Could you check a few things on this drawing? It's one solid part, dimensions in mm from its lowest x, y, z. Coordinates: 2 decimals unless noted, no trailing zeros. Write each loop counter-clockwise with the first axis right and the second up, starting at its lowest first coordinate (ties: lowest second). Pieces come first, ordered by that corner, then holes. Notation, with made-up numbers: (23, 16) - (38, 16) arc R23 cw to (38, 36) - close; hole circle Ø5 at (0, 58.5). An arc over 180 degrees is marked (long way). Answer as a JSON object with one key per item and string values. Group by question number.
1) If we section it at D-D (x = 12.75): Write out the boundary of the cut face in (y, z), plus the area to 3 significant figures.
2) Please list where these lines run through material, in increasing order: line 1 along Y through (x, z) = (4, 1.15); line 2 along Z through (x, y) = (3, 0.95); line 3 along Z through (x, y) = (6.75, 12).
3) If we section it at A-A (z = 26): Write out the boundary of the cut face in (x, y), plus the area to 3 significant figures.
4) If we section it at C-C (x = 4): Write out the boundary of the cut face in (y, z), plus the area to 3 significant figures.
5) Will these pins go through, and if not, where does the flat tip stop? pin 1 Ø2.5 at (x, y) = (16, 16) entering from +Z; pin 2 Ø5 at (x, z) = (13.5, 12) entering from -Y; pin 3 Ø10 at (x, z) = (13.5, 14.5) entering from +Y; pin 4 Ø9 at (x, y) = (9, 10.5) entering from +Z.
6) We'd pull the mould along Z, two halves only. Please class the marked faces 1, 2 and 3: released by +Z, released by -Z, zero draft, split by the parting line, or undercut.
7) If we section it at B-B (y = 6): Write out the boundary of the cut face in (x, z), plus the area to 3 significant figures.
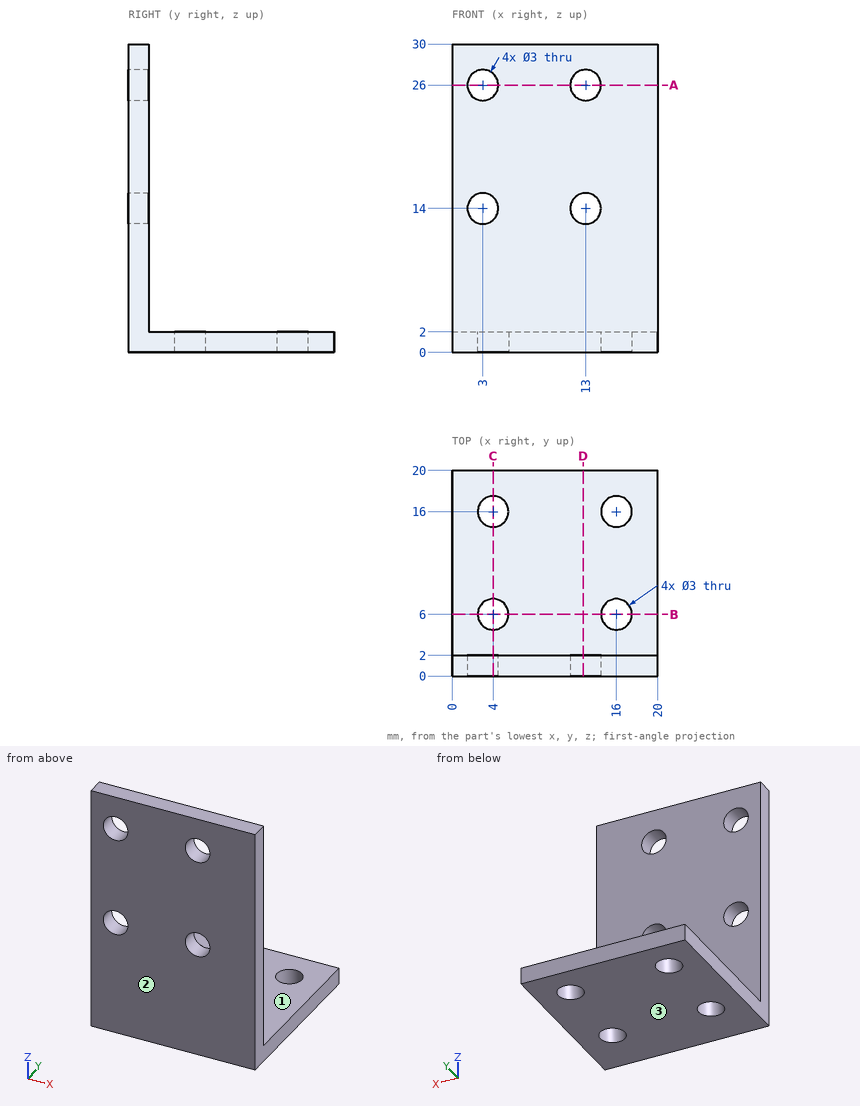
Here are the results:
{
 "1": {"outline": "(0, 0) - (20, 0) - (20, 2) - (2, 2) - (2, 12.52) - (0, 12.52) - close; (0, 15.48) - (2, 15.48) - (2, 24.52) - (0, 24.52) - close; (0, 27.48) - (2, 27.48) - (2, 30) - (0, 30) - close", "area": "84.2 mm²"},
 "2": {"line 1": "y = 0 to 4.5, 7.5 to 14.5, 17.5 to 20", "line 2": "z = 0 to 12.5, 15.5 to 24.5, 27.5 to 30", "line 3": "z = 0 to 2"},
 "3": {"outline": "(0, 0) - (1.5, 0) - (1.5, 2) - (0, 2) - close; (4.5, 0) - (11.5, 0) - (11.5, 2) - (4.5, 2) - close; (14.5, 0) - (20, 0) - (20, 2) - (14.5, 2) - close", "area": "28.0 mm²"},
 "4": {"outline": "(0, 0) - (4.5, 0) - (4.5, 2) - (2, 2) - (2, 12.88) - (0, 12.88) - close; (0, 15.12) - (2, 15.12) - (2, 24.88) - (0, 24.88) - close; (0, 27.12) - (2, 27.12) - (2, 30) - (0, 30) - close; (7.5, 0) - (14.5, 0) - (14.5, 2) - (7.5, 2) - close; (17.5, 0) - (20, 0) - (20, 2) - (17.5, 2) - close", "area": "75.1 mm²"},
 "5": {"pin 1": "passes through", "pin 2": "stops at y = 0", "pin 3": "stops at y = 2", "pin 4": "stops at z = 2"},
 "6": {"face 1": "released by +Z", "face 2": "zero draft", "face 3": "released by -Z"},
 "7": {"outline": "(0, 0) - (2.5, 0) - (2.5, 2) - (0, 2) - close; (5.5, 0) - (14.5, 0) - (14.5, 2) - (5.5, 2) - close; (17.5, 0) - (20, 0) - (20, 2) - (17.5, 2) - close", "area": "28.0 mm²"}
}
